Check sheet for the drawn part. Datum: minimum x, y, z corner. Units: mm. A direction names the side the tool comes from. Round coordinates to 2 decimals unless told otherwise and drop trailing zeros. Write each loop counter-clockwise with the first axis right and the second up, starting at its lowest first coordinate (ties: lowest second). Pieces come first, ordered by that corner, then holes. Notation, with made-up numbers: M 0.25,50 L 27.25,50 A19 ccw 27.25,57 Z; hole C 52.5,-3.5 d2. An arc over 180 degrees is marked long. Put each result on its own line as item: value.
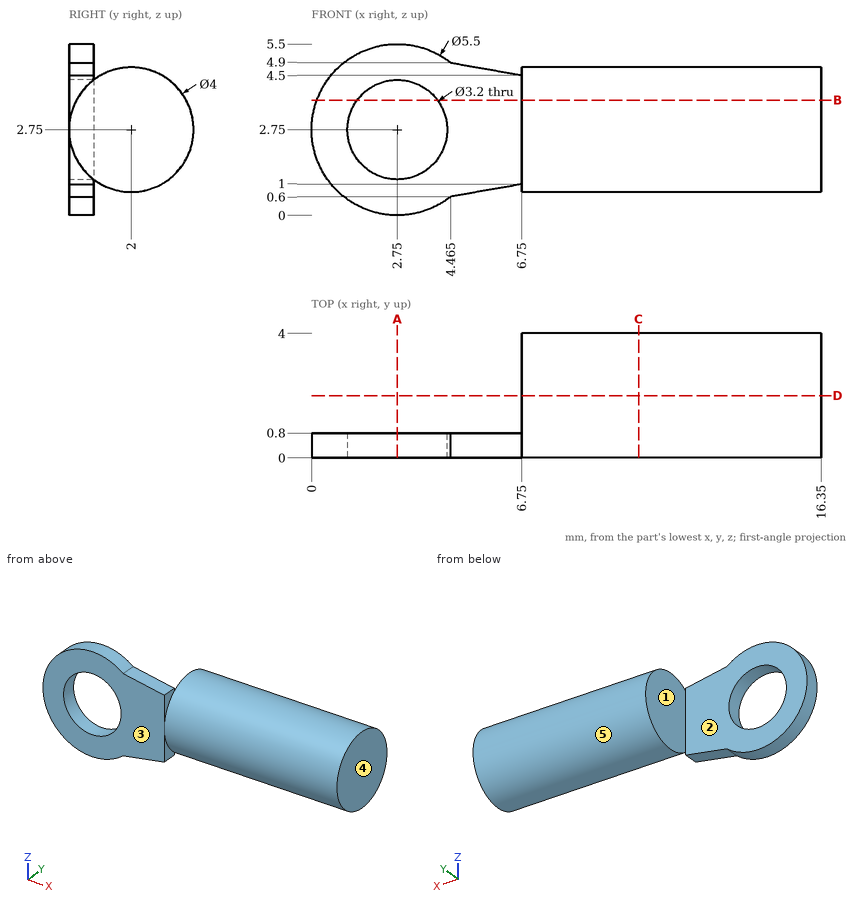
1. Release check for a two-part mould opening along Y. For the marked faces 1, 2 and 3 record: +Y half, -Y half, draft (parallel to the pull), parting line (faces both ways), or undercut.
Computed values:
face 1: draft
face 2: +Y half
face 3: -Y half
2. Depth check by flat-ended pin: pin 1 Ø3 at (x, z) = (2.75, 2.75) entering from +Y; pin 2 Ø1 at (x, y) = (13.5, 2.5) entering from +Z; pin 3 Ø2 at (x, z) = (10, 1) entering from +Y; pin 4 Ø1.7 at (x, z) = (5, 2.5) entering from +Y. Enter the tip coordinate at first touch or a pass-through.
Computed values:
pin 1: passes through
pin 2: stops at z = 4.75
pin 3: stops at y = 3.85
pin 4: stops at y = 0.8
3. Cross-section at B-B (z = 3.7). Enter the section's corners in (x, y), then the cut area to 3 significant figures.
Computed values:
outline: M 0.17,0 L 1.46,0 L 1.46,0.8 L 0.17,0.8 Z; M 4.04,0 L 6.75,0 L 6.75,0.24 L 16.35,0.24 L 16.35,3.76 L 6.75,3.76 L 6.75,0.8 L 4.04,0.8 Z
area: 37.0 mm2
4. Cross-section at C-C (x = 10.5). Enter the section's corners in (y, z).
Computed values:
outline: C 2,2.75 d4
5. Access from +Z, -Z, +X, -X, +Y, -Y to the whole of each face (thin tool, end or side, straight path). Record for the marked faces 4 and 5.
Computed values:
face 4: +Z, -Z, +X, +Y, -Y
face 5: +X
6. Scan lines: probe 1 along Z at (x, y) = (2.75, 0.4); probe 2 along X at (y, z) = (3.3, 2.3); probe 3 along Y at (x, z) = (4.5, 2). Record each from-to range of solid material in increasing order.
Computed values:
probe 1: z = 0 to 1.15, 4.35 to 5.5
probe 2: x = 6.75 to 16.35
probe 3: y = 0 to 0.8
7. Cross-section at D-D (y = 2). Enter the section's corners in (x, z).
Computed values:
outline: M 6.75,0.75 L 16.35,0.75 L 16.35,4.75 L 6.75,4.75 Z
8. Cross-section at A-A (x = 2.75). Enter the section's corners in (y, z).
Computed values:
outline: M 0,0 L 0.8,0 L 0.8,1.15 L 0,1.15 Z; M 0,4.35 L 0.8,4.35 L 0.8,5.5 L 0,5.5 Z
